Build history of the part. All positions in model axes, mm. A direction names the side the tool comes from. Give positions to 0.01 mm unless a question says otherwise; leave off trailing zeros. Loops run counter-clockwise (first coordinate to the right, second up) from the corner with the lowest first, then second, coordinate; pieces in that order, holes last. Notation, with made-up numbers: M 73,48 L 113,48 A21 cw 113,82 Z; hole C 44.25,4 d11. An arc over 180 degrees is marked long. Answer as a JSON object with one key per item and string values. Group by question number.
1. Mould opens along Y. For faces 1 (the face through (39, 50.8, 25)), 2 (the face through (323.73, 28.99, 25.04)), 3 (the face through (131, 37, 50.8)) say: released by +Y, released by -Y, zero draft, split by the parting line, or undercut.
2. Slice it at D-D (x = 290). List the corners of the cut face in (y, z).
3. Drill centre lines: line 1 along Y through (x, z) = (207.5, 7) (3 decimals); line 2 along Y through (x, z) = (284.5, 32) (3 decimals); line 3 along X through (y, z) = (21, 37.5). Where is each one in solid material? Low to high. Write a range as [from, to].
4. Slice it at C-C (y = 42.5). List the corners of the cut face in (x, z).
5. 3-axis set-ups, long thin cutter, end or side, ignore diameter. For faces 4 (the face through (76.2, 25, 25)), 5 (the face through (204.98, 44.36, 25.04)): which of +Z, -Z, +X, -X, +Y, -Y reach the whole face in a straight line?
6. Slice it at A-A (z = 8.5). List the corners of the cut face in (x, y).
7. Slice it at B-B (x = 116.5). List the corners of the cut face in (y, z) (3 decimals), then the cut area to 3 significant figures.
8. Drop flat-ended pins along their axis: pin 1 Ø12 at (y, z) = (6.5, 7) entering from -X; pin 2 Ø4 at (x, z) = (130, 25) entering from +Y; pin 3 Ø8 at (x, z) = (280.5, 43) entering from -Y (3 decimals); pin 4 Ø6 at (y, z) = (34.5, 5.5) entering from +X. Give the stop position or say it passes through.
from build123d import *

# Parameters (mm, degrees)
F1_DEPTH = 50.8
F3_DEPTH = 25.4
F5_DEPTH = 25.4


with BuildPart() as f1:
    # F0 (on Top) → F1 (new body)
    with BuildSketch(Plane.XY):
        Polygon((0, 50.8), (0, 0), (76.2, 0), (330.2, 12.7), (342.9, 25.4), (330.2, 38.1), (76.2, 50.8), align=None)
        Polygon((76.2, 12.7), (76.2, 38.1), (317.434589, 32.481896), (330.2, 25.4), (317.434589, 18.318104), align=None, mode=Mode.SUBTRACT)
    extrude(amount=F1_DEPTH)

    # F2 (on face) → F3 (join)
    with BuildSketch(Plane.XY.offset(50.8)):
        Polygon((330.2, 38.1), (76.2, 50.8), (76.2, 38.1), (317.434589, 32.481896), (330.2, 25.4), (317.434589, 18.318104), (76.2, 12.7), (76.2, 0), (330.2, 12.7), (342.9, 25.4), align=None)
    extrude(amount=-F3_DEPTH)

    # F4 (on face) → F5 (join)
    with BuildSketch(Plane.XY.offset(50.8)):
        Polygon((330.2, 38.1), (76.2, 50.8), (76.2, 38.1), (317.434589, 32.481896), (330.2, 25.4), (317.434589, 18.318104), (76.2, 12.7), (76.2, 0), (330.2, 12.7), (342.9, 25.4), align=None)
    extrude(amount=-F5_DEPTH)


solid = f1.part
Established:
{
 "1": {"face 1": "released by +Y", "face 2": "undercut", "face 3": "zero draft"},
 "2": {"outline": "M 10.69,0 L 17.68,0 L 17.68,50.8 L 10.69,50.8 Z; M 33.12,0 L 40.11,0 L 40.11,50.8 L 33.12,50.8 Z"},
 "3": {"line 1": "y = [6.565, 15.758], [35.042, 44.235]", "line 2": "y = [10.415, 17.551], [33.249, 40.385]", "line 3": "x = [0, 76.2], [322.27, 338.5]"},
 "4": {"outline": "M 0,0 L 242.2,0 L 242.2,50.8 L 0,50.8 Z"},
 "5": {"face 4": "+Z, -Z", "face 5": "+Z, -Z, +X, +Y"},
 "6": {"outline": "M 0,0 L 76.2,0 L 330.2,12.7 L 342.9,25.4 L 330.2,38.1 L 76.2,50.8 L 0,50.8 Z; hole M 76.2,12.7 L 317.43,18.32 L 330.2,25.4 L 317.43,32.48 L 76.2,38.1 Z"},
 "7": {"outline": "M 2.015,0 L 13.639,0 L 13.639,50.8 L 2.015,50.8 Z; M 37.161,0 L 48.785,0 L 48.785,50.8 L 37.161,50.8 Z", "area": "1,180 mm^2"},
 "8": {"pin 1": "stops at x = 0", "pin 2": "stops at y = 48.21", "pin 3": "stops at y = 10.015", "pin 4": "stops at x = 336.8"}
}
